For this review, take the finished solid that the model builds, in its own axes (mm). Face numbers are marked on the shaded views. A direction names the side the tool comes from. Give positions to 0.01 mm unless a question says otherwise; leave off trailing zeros. Loops run counter-clockwise (first coordinate to the right, second up) from the corner with the lowest first, then second, coordinate; pieces in that order, holes last. Notation, with made-up numbers: (6.5, 67) -> (57.5, 67) arc R13 ccw to (57.5, 86) -> close; hole circle Ø5 at (-3, -19.75). An arc over 180 degrees is marked (long way). One line per question, with ' | ' between items. Start each with the question number.
(1) Insertion check: P1, Ø1.5, axis at y = 13.5, z = 12, coming from the +X side; P2, Ø0.8, axis at x = 25.5, y = 13.5, coming from the -Z side. Each pin has a flat end and moves straight along its axis. Give the tip position at first contact, or say it passes through.
(2) Consider section C-C (x = 25.5). Write out the cut boundary in (y, z), and give its area (3 significant figures).
(3) Tool access review of the marked faces 1, 2, 3 and 4: name each direction out of +Z, -Z, +X, -X, +Y, -Y from which nothing blocks a thin tool from reaching the whole face with its end or side.
(4) Draft analysis for pull direction X (two halves, no side actions). For the marked faces 5, 6, 7 and 8, state which applies: +X half, -X half, draft (parallel to the pull), parting line (faces both ways), or undercut.
(5) Wall thickness on probe 1 along X at (y, z) = (14.25, 11.7); probe 2 along X at (y, z) = (13.6, 10.95); probe 3 along Y at (x, z) = (23.5, 12.8): over which ranges is each line inside the solid? List them lowest first.
(6) Consider section A-A (z = 11.2). Write out the cut boundary in (x, y), and give its area (3 significant figures).
(7) Consider section B-B (y = 13.95). Write out the cut boundary in (x, z).
(8) Consider section D-D (z = 10.3). Write out the cut boundary in (x, y), and give its area (3 significant figures).
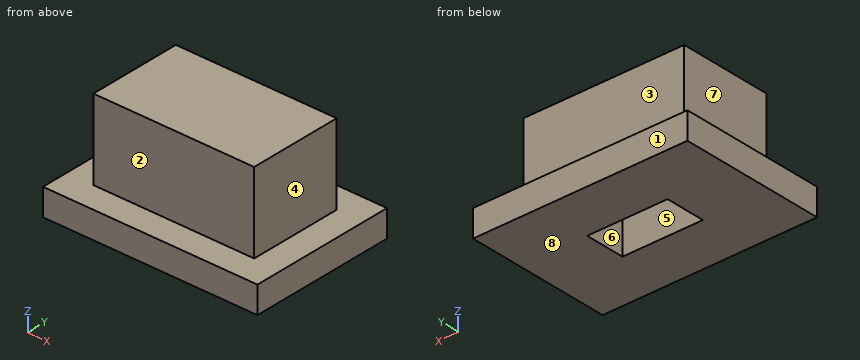
from build123d import *

# Parameters (mm, degrees)
BOX017_W     = 3
BOX017_H     = 1.5
BOX017_DEPTH = 2
BOX016_W     = 8
BOX016_H     = 5.5
BOX016_DEPTH = 1
BOX015_W     = 6
BOX015_H     = 3.5
BOX015_DEPTH = 3


with BuildPart() as cube015:
    # Box017 → Box017 (new body)
    with BuildSketch(Plane(origin=(23.5, 13, 10), x_dir=(1, 0, 0), z_dir=(0, 0, 1))):
        with Locations((1.5, 0.75)):
            Rectangle(BOX017_W, BOX017_H)
    extrude(amount=BOX017_DEPTH)


with BuildPart() as cube014:
    # Box016 → Box016 (new body)
    with BuildSketch(Plane(origin=(21, 11, 10), x_dir=(1, 0, 0), z_dir=(0, 0, 1))):
        with Locations((4, 2.75)):
            Rectangle(BOX016_W, BOX016_H)
    extrude(amount=BOX016_DEPTH)


with BuildPart() as obj1:
    # Box015 → Box015 (new body)
    with BuildSketch(Plane(origin=(22, 12, 11), x_dir=(1, 0, 0), z_dir=(0, 0, 1))):
        with Locations((3, 1.75)):
            Rectangle(BOX015_W, BOX015_H)
    extrude(amount=BOX015_DEPTH)

    # Fusion004: union Cube014
    add(cube014.part)

    # Cut004: cut Cube015
    add(cube015.part, mode=Mode.SUBTRACT)


solid = obj1.part
A:
1) P1: stops at x = 28 | P2: stops at z = 12
2) outline: (11, 10) -> (13, 10) -> (13, 12) -> (14.5, 12) -> (14.5, 10) -> (16.5, 10) -> (16.5, 11) -> (15.5, 11) -> (15.5, 14) -> (12, 14) -> (12, 11) -> (11, 11) -> close | area: 13.0 mm^2
3) face 1: +Z, -Z, +X, -X, +Y | face 2: +Z, +X, -X, -Y | face 3: +Z, +X, -X, +Y | face 4: +Z, +X, +Y, -Y
4) face 5: undercut | face 6: undercut | face 7: -X half | face 8: draft
5) probe 1: x = 22 to 23.5, 26.5 to 28 | probe 2: x = 21 to 23.5, 26.5 to 29 | probe 3: y = 12 to 15.5
6) outline: (22, 12) -> (28, 12) -> (28, 15.5) -> (22, 15.5) -> close; hole (23.5, 13) -> (26.5, 13) -> (26.5, 14.5) -> (23.5, 14.5) -> close | area: 16.5 mm^2
7) outline: (21, 10) -> (23.5, 10) -> (23.5, 12) -> (26.5, 12) -> (26.5, 10) -> (29, 10) -> (29, 11) -> (28, 11) -> (28, 14) -> (22, 14) -> (22, 11) -> (21, 11) -> close
8) outline: (21, 11) -> (29, 11) -> (29, 16.5) -> (21, 16.5) -> close; hole (23.5, 13) -> (26.5, 13) -> (26.5, 14.5) -> (23.5, 14.5) -> close | area: 39.5 mm^2
